Model file for the job. Use its own axes, mm. A direction names the side the tool comes from. Coordinates: 2 decimals unless noted, no trailing zeros. Order: outer loops, then holes, each group sorted by start corner. A loop starts at its lowest first (then second) coordinate and runs counter-clockwise, first axis right, second up. Notation, with made-up numbers: (87, -8.5) -> (109, -8.5) arc R15 cw to (109, 7.5) -> close; hole circle Ø11 at (19.5, -14.5). An arc over 180 degrees is marked (long way). Use CSV: the item, a comma, the result in double quotes. Start each with the question number.
(1) Pin check, flat tips, straight feed: pin 1 Ø2 at (x, z) = (-9.5, 0) entering from -Y; pin 2 Ø3 at (x, y) = (-1, 3.5) entering from -Z; pin 3 Ø2.5 at (x, z) = (9.5, 0) entering from +Y; pin 4 Ø3 at (y, z) = (3.5, -1) entering from +X. Stop position of each tip, or through.
(2) Cut at A-A on x = 0. Write the cut outline in (y, z), plus the area to 3 significant figures.
(3) Tool access for faces 5 (the flat face through (-11, 8, 1.2)), 6 (the cylindrical face through (7.84, 9.01, -0.37)), 7 (the cylindrical face through (-9.66, -1.52, 0.37)), 8 (the flat face through (-2, 0, -7)), 9 (the flat face through (1, 3, 5)): list every direction of +Z, -Z, +X, -X, +Y, -Y with a clear straight run to the whole face (end or side of a thin tool).
(4) Cut at D-D on z = 8. Write the cut outline in (x, y), plus the area to 3 significant figures.
(5) Pull direction Y, two halves, no side cores. Call faces 1 (the flat face through (5, 2, 0)), 2 (the flat face through (1, 3, -5)), 3 (the flat face through (7, 10, 0)), 4 (the flat face through (11.1, 8, -1)): pulls with the +Y half, pulls with the -Y half, needs draft (parallel to the pull), parting line crosses it, or undercut.
(6) Cut at C-C on y = 7. Write the cut outline in (x, z).
(7) Probe L1, parallel to X at y = -1.35, z = 0; L2, parallel to Z at x = -9.5, y = 8.95; L3, parallel to Y at x = -9.75, z = 3.5. List the from-to ranges inside material, lowest first.
(8) Cut at B-B on z = 0. Give the number of separate pieces and of enclosed holes in the cut face, plus the area to 3 significant figures.
```python
from build123d import *

# Parameters (mm, degrees)
EXTRUDE_1_DEPTH     = 5
SKETCH_2_R          = 11
EXTRUDE_2_DEPTH     = 3
SKETCH_3_R          = 1.7
CUT_EXTRUDE_1_DEPTH = 3
FILLET_1_R          = 0.5
CUT_EXTRUDE_2_REACH = 23.125
SKETCH_4_R          = 1.7


with BuildPart() as part:
    # 草图1 → 凸台-拉伸1 (new, symmetric)
    with BuildSketch(Plane.XY):
        with BuildLine():
            Line((5, 0), (-5, 0))
            Line((-5, 0), (-5, 4.409830056))
            ThreePointArc((-5, 4.409830056), (-6.372273568, 6.044733944), (-7.228416147, 8))
            Line((-7.228416147, 8), (-12.5, 8))
            Line((-12.5, 8), (-12.5, 10))
            Line((-12.5, 10), (-6.5, 10))
            ThreePointArc((-6.5, 10), (0, 3.5), (6.5, 10))
            Line((6.5, 10), (12.5, 10))
            Line((12.5, 10), (12.5, 8))
            Line((12.5, 8), (7.228416147, 8))
            ThreePointArc((7.228416147, 8), (6.372273568, 6.044733944), (5, 4.409830056))
            Line((5, 4.409830056), (5, 0))
        make_face()
    extrude(amount=EXTRUDE_1_DEPTH, both=True)

    # 草图2 → 凸台-拉伸2 (add)
    with BuildSketch(Plane.XZ):
        with Locations(Location((0, 0, 0), (0, 0, 270))):
            Circle(SKETCH_2_R)
    extrude(amount=EXTRUDE_2_DEPTH)

    # 草图3 → 切除-拉伸1 (cut)
    with BuildSketch(Plane.XZ.offset(3)):
        with Locations(Location((0, 8, 0), (0, 0, 270))):
            Circle(SKETCH_3_R)
        with Locations(Location((8, 0, 0), (0, 0, 270))):
            Circle(SKETCH_3_R)
        with Locations(Location((0, -8, 0), (0, 0, 270))):
            Circle(SKETCH_3_R)
        with Locations(Location((-8, 0, 0), (0, 0, 270))):
            Circle(SKETCH_3_R)
    extrude(amount=-CUT_EXTRUDE_1_DEPTH, mode=Mode.SUBTRACT)

    # 圆角1
    fillet_1_edges = [part.edges().sort_by_distance(p)[0] for p in [
        (0, 0, -5),
        (5, 0, 0),
        (-5, 0, 0),
        (0, 0, 5),
    ]]
    fillet(fillet_1_edges, radius=FILLET_1_R)

    # 草图4 → 切除-拉伸2 (cut, up to next)
    with BuildSketch(Plane(origin=(0, 10, 0), x_dir=(1, 0, 0), z_dir=(0, 1, 0)), mode=Mode.PRIVATE) as cut_extrude_2_sk1:
        with Locations(Location((-9.5, 0, 0), (0, 0, 180))):
            Circle(SKETCH_4_R)
    cut_extrude_2_tool1 = extrude(cut_extrude_2_sk1.sketch, amount=-CUT_EXTRUDE_2_REACH, mode=Mode.PRIVATE) & part.part
    # 草图4 → 切除-拉伸2 (cut, up to next)
    with BuildSketch(Plane(origin=(0, 10, 0), x_dir=(1, 0, 0), z_dir=(0, 1, 0)), mode=Mode.PRIVATE) as cut_extrude_2_sk2:
        with Locations(Location((9.5, 0, 0), (0, 0, 270))):
            Circle(SKETCH_4_R)
    cut_extrude_2_tool2 = extrude(cut_extrude_2_sk2.sketch, amount=-CUT_EXTRUDE_2_REACH, mode=Mode.PRIVATE) & part.part
    add(cut_extrude_2_tool1.solids().sort_by_distance((-9.5, 10, 0))[0], mode=Mode.SUBTRACT)
    add(cut_extrude_2_tool2.solids().sort_by_distance((9.5, 10, 0))[0], mode=Mode.SUBTRACT)


solid = part.part
```
Outcome:
1,pin 1,"y = -3"
1,pin 2,"z = -5"
1,pin 3,"y = 0"
1,pin 4,"x = 5.59"
2,outline,"(-3, -11) -> (0, -11) -> (0, -9.7) -> (-3, -9.7) -> close; (-3, -6.3) -> (0, -6.3) -> (0, -5.5) arc R0.5 cw to (0.5, -5) -> (3.5, -5) -> (3.5, 5) -> (0.5, 5) arc R0.5 cw to (0, 5.5) -> (0, 6.3) -> (-3, 6.3) -> close; (-3, 9.7) -> (0, 9.7) -> (0, 11) -> (-3, 11) -> close"
2,area,"80.7 mm2"
3,face 5,"+Z, -Z, -X"
3,face 6,"+Y"
3,face 7,"-Y"
3,face 8,"none"
3,face 9,"+Z, +X, -X, +Y"
4,outline,"(-7.55, -3) -> (-1.7, -3) -> (-1.7, 0) -> (-7.55, 0) -> close; (1.7, -3) -> (7.55, -3) -> (7.55, 0) -> (1.7, 0) -> close"
4,area,"35.1 mm2"
5,face 1,"undercut"
5,face 2,"needs draft"
5,face 3,"pulls with the +Y half"
5,face 4,"undercut"
6,outline,"(-6.87, -5) -> (-5.77, -5) -> (-5.77, 5) -> (-6.87, 5) -> close; (5.77, -5) -> (6.87, -5) -> (6.87, 5) -> (5.77, 5) -> close"
7,L1,"-11 to -9.7, -6.3 to 6.3, 9.7 to 11"
7,L2,"-5 to -1.7, 1.7 to 5"
7,L3,"-3 to 0, 8 to 10"
8,separate pieces,"5"
8,enclosed holes,"0"
8,area,"105 mm2"
